```python
from build123d import *

# Parameters (mm, degrees)
F0_W        = 80
F0_H        = 144.526
F1_DEPTH    = 18.5
F2_T        = -2.5
F3_T1_DEPTH = 169.526
F3_T3_DEPTH = 43.5


# Not quite as in the source:
# - a fillet or chamfer that OpenCascade refuses, or shapes differently, is made with other operations: its cross-section is extruded or revolved along the edge and cut away or added


with BuildPart() as f1:
    # F0 (on Front) → F1 (new body)
    with BuildSketch(Plane.XZ):
        with Locations((4.5181000233, 3.1507380013)):
            Rectangle(F0_W, F0_H)
    extrude(amount=F1_DEPTH)

    # F2
    f2_openings = [f1.faces().sort_by_distance(p)[0] for p in [
        (4.5181, -9.25, 75.413738),
    ]]
    offset(amount=F2_T, openings=f2_openings)

    # F3: fillet of radius 5 on 8 edges, made by hand

    # F3_s2 → F3_t1 (cut)
    with BuildSketch(Plane.XY.offset(-81.6122619987)):
        with BuildLine():
            ThreePointArc((-35.4818999767, -13.5), (-34.0174338827, -17.0355339059), (-30.4818999767, -18.5))
            Line((-30.4818999767, -18.5), (-35.4818999767, -18.5))
            Line((-35.4818999767, -18.5), (-35.4818999767, -13.5))
        make_face()
        with BuildLine():
            ThreePointArc((-35.4818999767, -5), (-34.0174338827, -1.4644660941), (-30.4818999767, 0))
            Line((-30.4818999767, 0), (-35.4818999767, 0))
            Line((-35.4818999767, 0), (-35.4818999767, -5))
        make_face()
        with BuildLine():
            ThreePointArc((44.5181000233, -13.5), (43.0536339292, -17.0355339059), (39.5181000233, -18.5))
            Line((39.5181000233, -18.5), (44.5181000233, -18.5))
            Line((44.5181000233, -18.5), (44.5181000233, -13.5))
        make_face()
        with BuildLine():
            ThreePointArc((44.5181000233, -5), (43.0536339292, -1.4644660941), (39.5181000233, 0))
            Line((39.5181000233, 0), (44.5181000233, 0))
            Line((44.5181000233, 0), (44.5181000233, -5))
        make_face()
    extrude(amount=F3_T1_DEPTH, mode=Mode.SUBTRACT)

    # F3_s4 → F3_t3 (cut)
    with BuildSketch(Plane.XZ.offset(-12.5)):
        with BuildLine():
            ThreePointArc((44.5181000233, 70.4137380013), (43.0536339292, 73.9492719073), (39.5181000233, 75.4137380013))
            Line((39.5181000233, 75.4137380013), (44.5181000233, 75.4137380013))
            Line((44.5181000233, 75.4137380013), (44.5181000233, 70.4137380013))
        make_face()
        with BuildLine():
            ThreePointArc((-35.4818999767, 70.4137380013), (-34.0174338827, 73.9492719073), (-30.4818999767, 75.4137380013))
            Line((-30.4818999767, 75.4137380013), (-35.4818999767, 75.4137380013))
            Line((-35.4818999767, 75.4137380013), (-35.4818999767, 70.4137380013))
        make_face()
        with BuildLine():
            ThreePointArc((-35.4818999767, -64.1122619987), (-34.0174338827, -67.6477959046), (-30.4818999767, -69.1122619987))
            Line((-30.4818999767, -69.1122619987), (-35.4818999767, -69.1122619987))
            Line((-35.4818999767, -69.1122619987), (-35.4818999767, -64.1122619987))
        make_face()
        with BuildLine():
            ThreePointArc((39.5181000233, -69.1122619987), (43.0536339292, -67.6477959046), (44.5181000233, -64.1122619987))
            Line((44.5181000233, -64.1122619987), (44.5181000233, -69.1122619987))
            Line((44.5181000233, -69.1122619987), (39.5181000233, -69.1122619987))
        make_face()
    extrude(amount=F3_T3_DEPTH, mode=Mode.SUBTRACT)


solid = f1.part
```
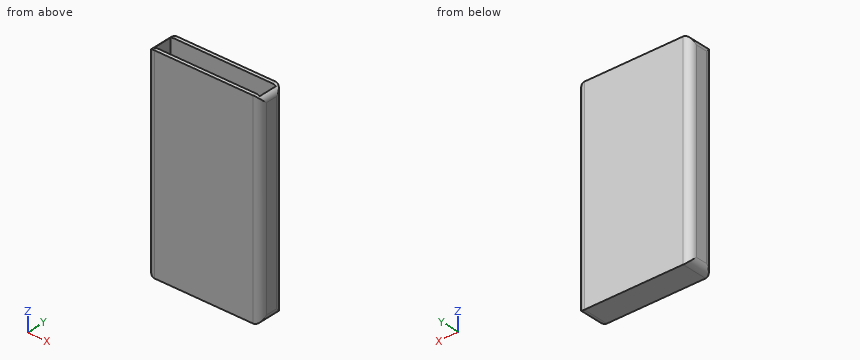
Could you check a few things on this model? Use its own coordinates, in mm. Give positions to 0.01 mm unless a question says otherwise; leave off trailing zeros. Loops run counter-clockwise (first coordinate to the right, second up) from the corner with the lowest first, then second, coordinate; pieces in that order, holes last. Notation, with made-up numbers: (28.25, -25) - (87.25, -25) arc R19 cw to (87.25, 7) - close; hole circle Ø11 at (84, -36). An arc over 180 degrees is marked (long way). Answer in a Markdown table with one row per item. Add a question column.
Q1. Please list where these lines run through material, in increasing order: L1, parallel to X at y = -11, z = -39; L2, parallel to Y at x = 17, z = -7; L3, parallel to Z at x = -10, y = -6.75. Write a range as from..to.
Q2. If we section it at C-C (x = 30): List the corners of the cut face in (y, z) for me, plus the area to 3 significant figures.
Q3. If we section it at B-B (y = -10.75): List the corners of the cut face in (x, z) for me.
Q4. If we section it at A-A (z = 54): List the corners of the cut face in (x, y) for me.
The answers:
| question | item | result |
|---|---|---|
| 1 | L1 | x = -35.48..-32.98, 42.02..44.52 |
| 1 | L2 | y = -18.5..-16, -2.5..0 |
| 1 | L3 | z = -69.11..-66.61 |
| 2 | outline | (-18.5, -69.11) - (0, -69.11) - (0, 75.41) - (-2.5, 75.41) - (-2.5, -66.61) - (-16, -66.61) - (-16, 75.41) - (-18.5, 75.41) - close |
| 2 | area | 756 mm^2 |
| 3 | outline | (-35.48, -64.11) arc R5 ccw to (-30.48, -69.11) - (39.52, -69.11) arc R5 ccw to (44.52, -64.11) - (44.52, 70.41) arc R5 ccw to (42.02, 74.74) - (42.02, -66.61) - (-32.98, -66.61) - (-32.98, 74.74) arc R5 ccw to (-35.48, 70.41) - close |
| 4 | outline | (-35.48, -13.5) arc R5 ccw to (-30.48, -18.5) - (39.52, -18.5) arc R5 ccw to (44.52, -13.5) - (44.52, -5) arc R5 ccw to (39.52, 0) - (-30.48, 0) arc R5 ccw to (-35.48, -5) - close; hole (-32.98, -16) - (42.02, -16) - (42.02, -2.5) - (-32.98, -2.5) - close |
